Geometry check sheet. Reference: the model listing, model coordinates, mm. Give positions to 0.01 mm unless a question says otherwise; leave off trailing zeros. Use a Markdown table: item, result. Add a question column.
1. Cross-section at A-A on x = -0.7. Count the separate pieces of the cut face and the enclosed holes in it, and give its area (3 significant figures).
2. Material ranges on L1, parallel to Z at x = 0.2, y = -68.75; L2, parallel to Z at x = 0.35, y = -81.25 (3 decimals); L3, parallel to Y at x = -0.5, z = -0.25, recorded low to high.
3. Depth check by flat-ended pin: P1, Ø1.9, axis at y = -51.25, z = -4, coming from the +X side; P2, Ø1, axis at x = 0, y = -89.5, coming from the +Z side (3 decimals). Enter the tip coordinate at first touch or a pass-through.
from build123d import *

# Parameters (mm, degrees)
SKETCH_1_W           = 14
SKETCH_1_H           = 182.5
EXTRUDE_1_DEPTH      = 1
SKETCH_2_W           = 2.45
SKETCH_2_H           = 5
CUT_EXTRUDE_1_DEPTH  = 3
SKETCH_3_R           = 0.6
CUT_EXTRUDE_2_DEPTH  = 3
SKETCH_6_W           = 2.45
SKETCH_6_H           = 5
CUT_EXTRUDE_4_DEPTH  = 3
SKETCH_7_R           = 0.6
CUT_EXTRUDE_5_DEPTH  = 3
SKETCH_8_R           = 1.55
CUT_EXTRUDE_6_DEPTH  = 3
SKETCH_9_W           = 2.45
SKETCH_9_H           = 7
CUT_EXTRUDE_7_DEPTH  = 3
SKETCH_10_R          = 0.6
CUT_EXTRUDE_8_DEPTH  = 3
CUT_EXTRUDE_9_DEPTH  = 3
SKETCH_12_R          = 1.05
CUT_EXTRUDE_10_DEPTH = 3
SKETCH_14_R          = 1.05
CUT_EXTRUDE_11_DEPTH = 3
SKETCH_15_R          = 1.05
CUT_EXTRUDE_12_DEPTH = 3


with BuildPart() as part:
    # 草图1 → 凸台-拉伸1 (new body, symmetric)
    with BuildSketch(Plane(origin=(0, 0, 0), x_dir=(0, 0, -1), z_dir=(1, 0, 0))):
        Rectangle(SKETCH_1_W, SKETCH_1_H)
    extrude(amount=EXTRUDE_1_DEPTH, both=True)

    # 草图2 → 切除-拉伸1 (cut, through all)
    with BuildSketch(Plane(origin=(1, 0, 0), x_dir=(0, 0, -1), z_dir=(1, 0, 0))):
        with Locations((0, -88.75)):
            Rectangle(SKETCH_2_W, SKETCH_2_H)
    extrude(amount=-CUT_EXTRUDE_1_DEPTH, mode=Mode.SUBTRACT)

    # 草图3 → 切除-拉伸2 (cut, through all)
    with BuildSketch(Plane(origin=(1, 0, 0), x_dir=(0, 0, -1), z_dir=(1, 0, 0))):
        with Locations((-1.225, -86.85)):
            Circle(SKETCH_3_R)
        with Locations((1.225, -86.85)):
            Circle(SKETCH_3_R)
    extrude(amount=-CUT_EXTRUDE_2_DEPTH, mode=Mode.SUBTRACT)

    # 草图6 → 切除-拉伸4 (cut, through all)
    with BuildSketch(Plane(origin=(1, 0, 0), x_dir=(0, 0, -1), z_dir=(1, 0, 0))):
        with Locations((0, -73.7)):
            Rectangle(SKETCH_6_W, SKETCH_6_H)
    extrude(amount=-CUT_EXTRUDE_4_DEPTH, mode=Mode.SUBTRACT)

    # 草图7 → 切除-拉伸5 (cut, through all)
    with BuildSketch(Plane(origin=(1, 0, 0), x_dir=(0, 0, -1), z_dir=(1, 0, 0))):
        with Locations((-1.225, -71.8)):
            Circle(SKETCH_7_R)
        with Locations((-1.225, -75.6)):
            Circle(SKETCH_7_R)
        with Locations((1.225, -71.8)):
            Circle(SKETCH_7_R)
        with Locations((1.225, -75.6)):
            Circle(SKETCH_7_R)
    extrude(amount=-CUT_EXTRUDE_5_DEPTH, mode=Mode.SUBTRACT)

    # 草图8 → 切除-拉伸6 (cut, through all)
    with BuildSketch(Plane(origin=(1, 0, 0), x_dir=(0, 0, -1), z_dir=(1, 0, 0))):
        with Locations((-4.225, -81.25)):
            Circle(SKETCH_8_R)
        with Locations((4.225, -81.25)):
            Circle(SKETCH_8_R)
    extrude(amount=-CUT_EXTRUDE_6_DEPTH, mode=Mode.SUBTRACT)

    # 草图9 → 切除-拉伸7 (cut, through all)
    with BuildSketch(Plane(origin=(1, 0, 0), x_dir=(0, 0, -1), z_dir=(1, 0, 0))):
        with Locations((0, 81.25)):
            Rectangle(SKETCH_9_W, SKETCH_9_H)
    extrude(amount=-CUT_EXTRUDE_7_DEPTH, mode=Mode.SUBTRACT)

    # 草图10 → 切除-拉伸8 (cut, through all)
    with BuildSketch(Plane(origin=(1, 0, 0), x_dir=(0, 0, -1), z_dir=(1, 0, 0))):
        with Locations((-1.225, 84.15)):
            Circle(SKETCH_10_R)
        with Locations((-1.225, 78.35)):
            Circle(SKETCH_10_R)
        with Locations((1.225, 84.15)):
            Circle(SKETCH_10_R)
        with Locations((1.225, 78.35)):
            Circle(SKETCH_10_R)
    extrude(amount=-CUT_EXTRUDE_8_DEPTH, mode=Mode.SUBTRACT)

    # 草图11 → 切除-拉伸9 (cut, through all)
    with BuildSketch(Plane(origin=(1, 0, 0), x_dir=(0, 0, -1), z_dir=(1, 0, 0))):
        Polygon((-3, -91.25), (-7, -83.25), (-7, -91.25), align=None)
        Polygon((7, -83.25), (7, -91.25), (3, -91.25), align=None)
    extrude(amount=-CUT_EXTRUDE_9_DEPTH, mode=Mode.SUBTRACT)

    # 草图12 → 切除-拉伸10 (cut, through all)
    with BuildSketch(Plane(origin=(1, 0, 0), x_dir=(0, 0, -1), z_dir=(1, 0, 0))):
        with Locations((-4, -68.75)):
            Circle(SKETCH_12_R)
    extrude(amount=-CUT_EXTRUDE_10_DEPTH, mode=Mode.SUBTRACT)

    # 草图14 → 切除-拉伸11 (cut, through all)
    with BuildSketch(Plane.ZY.offset(1)):
        with Locations((-2.5, -68.75)):
            Circle(SKETCH_14_R)
    extrude(amount=-CUT_EXTRUDE_11_DEPTH, mode=Mode.SUBTRACT)

    # 草图15 → 切除-拉伸12 (cut, through all)
    with BuildSketch(Plane.ZY.offset(1)):
        with Locations((-4, -51.25)):
            Circle(SKETCH_15_R)
        with Locations((4, -51.25)):
            Circle(SKETCH_15_R)
    extrude(amount=-CUT_EXTRUDE_12_DEPTH, mode=Mode.SUBTRACT)


solid = part.part
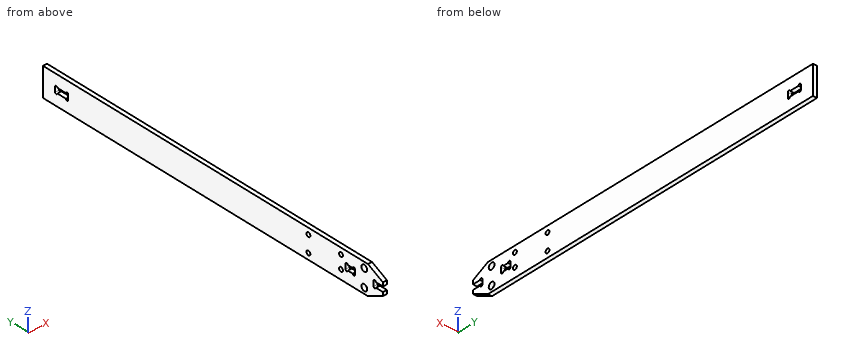
Values found:
| question | item | result |
|---|---|---|
| 1 | separate pieces | 1 |
| 1 | enclosed holes | 8 |
| 1 | area | 2,450 mm2 |
| 2 | L1 | z = -7 to -3.55, -1.45 to 2.95, 5.05 to 7 |
| 2 | L2 | z = -7 to -5.775, -2.675 to 2.675, 5.775 to 7 |
| 2 | L3 | y = -86.25 to -76.2, -71.2 to 77.75, 84.75 to 91.25 |
| 3 | P1 | passes through |
| 3 | P2 | stops at z = 4.125 |
